Work out the finished part from the listing and answer in its coordinate system (mm). A direction names the side the tool comes from. Round coordinates to 2 decimals unless told otherwise and drop trailing zeros. Loops run counter-clockwise (first coordinate to the right, second up) from the corner with the lowest first, then second, coordinate; pieces in that order, holes last. Notation, with made-up numbers: (26, 69) - (73, 69) arc R18 ccw to (73, 85) - close; hole circle Ø4 at (67.25, -2). An arc over 180 degrees is marked (long way). Answer as CSV lines item,"result". Start each with the question number.
Q1. Straight lines are drawn through the part: L1, parallel to X at y = 31, z = 47; L2, parallel to Z at x = -3, y = 10; L3, parallel to Y at x = -68, z = 26.5. For each, find the intervals that lie inside material, in ascending order. Write a range as [from, to].
Q2. The mould has two halves that part along Y. Classify faces 3 (the face through (-61, -33.254, 99)), 4 (the face through (30.993, 6, 99)), 5 (the face through (-61, 5, 0)): +Y half, -Y half, draft (parallel to the pull), parting line (faces both ways), or undercut.
Q3. Section A-A on x = -9 is taken. Write down the section's boundary in (y, z), then the cut area to 3 significant figures.
Q4. For faces 1 (the face through (-61, 42.746, 96)), 2 (the face through (-151.007, 6, 99)), determine the directions among +Z, -Z, +X, -X, +Y, -Y from which every point of the face is accessible in a straight line to the end or side of a thin tool.
Q5. Section B-B on z = 171 is taken. Write down the section's boundary in (x, y).
```python
from build123d import *

# Parameters (mm, degrees)
F0_W     = 182
F0_H     = 77
F0_W_2   = 180
F0_H_2   = 75
F1_DEPTH = 195
F2_W     = 182
F2_H     = 77
F2_W_2   = 180
F2_H_2   = 75
F3_DEPTH = 1
F4_W     = 182
F4_H     = 77
F4_W_2   = 180
F4_H_2   = 75
F5_DEPTH = 1


with BuildPart() as f1:
    # F0 (on Top) → F1 (new body)
    with BuildSketch(Plane.XY):
        with Locations((-60.0073022693, 5.2463471889)):
            Rectangle(F0_W, F0_H)
        with Locations((-60.0073022693, 5.2463471889)):
            Rectangle(F0_W_2, F0_H_2, mode=Mode.SUBTRACT)
    extrude(amount=F1_DEPTH)

    # F2 (on face) → F3 (join)
    with BuildSketch(Plane.XY.offset(195)):
        with Locations((-60.0073022693, 5.2463471889)):
            Rectangle(F2_W, F2_H)
        with Locations((-60.0073022693, 5.2463471889)):
            Rectangle(F2_W_2, F2_H_2, mode=Mode.SUBTRACT)
        with Locations((-60.0073022693, 5.2463471889)):
            Rectangle(F2_W_2, F2_H_2)
    extrude(amount=F3_DEPTH)

    # F4 (on face) → F5 (join)
    with BuildSketch(Plane(origin=(0, 0, 0), x_dir=(1, 0, 0), z_dir=(0, 0, -1))):
        with Locations((-60.0073022693, -5.2463471889)):
            Rectangle(F4_W, F4_H)
        with Locations((-60.0073022693, -5.2463471889)):
            Rectangle(F4_W_2, F4_H_2, mode=Mode.SUBTRACT)
        with Locations((-60.0073022693, -5.2463471889)):
            Rectangle(F4_W_2, F4_H_2)
    extrude(amount=F5_DEPTH)


solid = f1.part
```
Findings:
1,L1,"x = [-151.01, -150.01], [29.99, 30.99]"
1,L2,"z = [-1, 0], [195, 196]"
1,L3,"y = [-33.25, -32.25], [42.75, 43.75]"
2,face 3,"-Y half"
2,face 4,"draft"
2,face 5,"undercut"
3,outline,"(-33.25, -1) - (43.75, -1) - (43.75, 196) - (-33.25, 196) - close; hole (-32.25, 0) - (42.75, 0) - (42.75, 195) - (-32.25, 195) - close"
3,area,"544 mm^2"
4,face 1,"none"
4,face 2,"+Z, -Z, -X, +Y, -Y"
5,outline,"(-151.01, -33.25) - (30.99, -33.25) - (30.99, 43.75) - (-151.01, 43.75) - close; hole (-150.01, -32.25) - (29.99, -32.25) - (29.99, 42.75) - (-150.01, 42.75) - close"
